Could you check a few things on this model? Use its own coordinates, in mm. A direction names the side the tool comes from. Round coordinates to 2 decimals unless told otherwise and drop trailing zeros. Loops run counter-clockwise (first coordinate to the right, second up) from the corner with the lowest first, then second, coordinate; pieces in that order, holes last. Notation, with made-up numbers: (-3, -18) -> (11, -18) arc R33 cw to (11, 17) -> close; hole circle Ø4 at (-32.75, 89). An arc over 180 degrees is marked (long way). One line per item, written item: value.
Autodesk Inventor part; units mm, degrees
ref_plane "YZ Plane" through (0, 0, 0) normal (1, 0, 0) x (0, 1, 0)
ref_plane "XZ Plane" through (0, 0, 0) normal (0, 1, 0) x (-1, 0, 0)
ref_plane "XY Plane" through (0, 0, 0) normal (0, 0, 1) x (1, 0, 0)
sketch "Sketch1" plane through (0, 0, 0) normal (0, 1, 0) x (-1, 0, 0)
  circle A0 centre (0, 0) radius 25.4
  dimension "d0" = 50.8
extrude "Extrusion1" add sketch "Sketch1" along normal blind 17.78
shell "Shell1" thickness 1.27 removed faces 1 at (7.2508, 17.78, -1.9085)
sketch "Sketch2" plane through (0, 0, 0) normal (0, -1, 0) x (1, 0, 0)
  circle A0 centre (0, 0) radius 22.86
  dimension "d4" = 45.72
extrude "Extrusion2" cut sketch "Sketch2" against normal blind 7.62
sketch "Sketch4" plane through (0, 17.78, 0) normal (0, 1, 0) x (1, 0, 0)
  circle A0 centre (0, 0) radius 25.4
  circle A1 centre (0, 0) radius 24.13
extrude "Extrusion4" cut sketch "Sketch4" against normal blind 10.16
sketch "Sketch5" plane through (0, 1.27, 0) normal (0, 1, 0) x (1, 0, 0)
  circle A0 centre (0, 0) radius 23.7732
  circle A1 centre (0, 0) radius 22.86
extrude "Extrusion5" cut sketch "Sketch5" against normal blind 7.62
properties part number "Adapter"
(1) If we section it at C-C, the plane y = 3.75: Please give me the cut outline in (x, z).
Recorded:
outline: circle Ø50.8 at (0, 0); hole circle Ø48.26 at (0, 0)
(2) If we section it at A-A, the plane x = 0: Please give me the cut outline in (y, z).
Recorded:
outline: (0, -25.4) -> (7.62, -25.4) -> (7.62, -24.13) -> (1.27, -24.13) -> (1.27, -23.77) -> (0, -23.77) -> close; (0, 23.77) -> (1.27, 23.77) -> (1.27, 24.13) -> (7.62, 24.13) -> (7.62, 25.4) -> (0, 25.4) -> close
(3) Thinking about a two-plate mould opening in Z: for faces 3 (the face through (22.5, 7.62, 9.3)), 4 (the face through (-17.8, 1.27, -16)), 5 (the face through (5.506, 3.757, 24.796)), which applies, released by +Z, released by -Z, zero draft, split by the parting line, or undercut?
Recorded:
face 3: zero draft
face 4: undercut
face 5: split by the parting line
(4) I'm going to push flat-ended pins straight in: pin 1 Ø4 at (x, y) = (-7, 6) entering from +Z; pin 2 Ø24 at (x, z) = (-5.5, 8.5) entering from +Y; pin 3 Ø1 at (y, z) = (5.5, 16.5) entering from -X. Where does each tip first touch, or does it pass through?
Recorded:
pin 1: z = 24.9
pin 2: through
pin 3: x = -19.73
(5) If we section it at B-B, the plane z = -1: Please give me the cut outline in (x, y), then the cut area to 3 significant figures.
Recorded:
outline: (-25.38, 0) -> (-23.75, 0) -> (-23.75, 1.27) -> (-24.11, 1.27) -> (-24.11, 7.62) -> (-25.38, 7.62) -> close; (23.75, 0) -> (25.38, 0) -> (25.38, 7.62) -> (24.11, 7.62) -> (24.11, 1.27) -> (23.75, 1.27) -> close
area: 20.3 mm²
(6) If I drill on L1, parallel to Z at x = 0, y = 5.5; L2, parallel to X at y = 0.65, z = 0, over which ranges is the centre line in solid material (lowest first)?
Recorded:
L1: -25.4 to -24.13, 24.13 to 25.4
L2: -25.4 to -23.77, 23.77 to 25.4
(7) For faces 1 (the face through (-23.016, 4.401, -7.248)), 2 (the face through (22.675, 0.644, -7.141)), which set-ups out of +Z, -Z, +X, -X, +Y, -Y let a thin tool reach every point of the face, with its end or its side?
Recorded:
face 1: +Y
face 2: +Y, -Y
